The model under review builds one solid part; all positions refer to its coordinate system, in mm. A direction names the side the tool comes from. Round coordinates to 2 decimals unless told otherwise and drop trailing zeros. Loops run counter-clockwise (first coordinate to the right, second up) from the corner with the lowest first, then second, coordinate; pieces in that order, holes last. Notation, with made-up numbers: (59.25, -33) -> (112.25, -33) arc R24 cw to (112.25, -7) -> close; hole circle Ø7 at (13, -0.5). An arc over 180 degrees is marked (long way). Use a Markdown table: item, result. Add a question column.
1) Consider section A-A on x = 0. Give the boundary of the cut face in (y, z), plus the area to 3 significant figures.
2) Consider section C-C on z = -293.5. Give the boundary of the cut face in (x, y), plus the area to 3 significant figures.
3) For faces 1 (the cylindrical face through (23.517, -36.886, -300.533)), 2 (the flat face through (-4, -203.2, 100)), list the 3-axis set-ups (+Z, -Z, +X, -X, +Y, -Y) from which the entire face can be reached by the end or side of a thin tool; tool diameter is ignored.
4) Insertion check: pin 1 (12 mm diameter, centred on x = 137, y = 57, fed in from -Z). The pin has a flat end and moves straight along its axis. Give the tip position at first contact, or say it passes through.
5) Wall thickness on probe 1 along Z at (x, y) = (-12, 149); probe 2 along X at (y, z) = (-19.5, -450); probe 3 along Y at (x, z) = (-39.5, -228): over which ranges is each line inside the solid? List them lowest first.
6) Consider section D-D on y = 175. Give the boundary of the cut face in (x, z).
7) Consider section B-B on y = 0. Give the boundary of the cut face in (x, z).
from build123d import *

# Parameters (mm, degrees)
SKETCH_W     = 609.6
SKETCH_H     = 406.4
PAD_DEPTH    = 203.2
SKETCH001_R  = 43.745106
PAD001_DEPTH = 609.6


with BuildPart() as part:
    # Sketch → Pad (new body)
    with BuildSketch(Plane.XY):
        Rectangle(SKETCH_W, SKETCH_H)
    extrude(amount=PAD_DEPTH)

    # Sketch001 (on Face5 of Pad) → Pad001 (join)
    with BuildSketch(Plane(origin=(0, 0, 0), x_dir=(1, 0, 0), z_dir=(0, 0, -1))):
        Circle(SKETCH001_R)
    extrude(amount=PAD001_DEPTH)


solid = part.part
Result set:
| question | item | result |
|---|---|---|
| 1 | outline | (-203.2, 0) -> (-43.75, 0) -> (-43.75, -609.6) -> (43.75, -609.6) -> (43.75, 0) -> (203.2, 0) -> (203.2, 203.2) -> (-203.2, 203.2) -> close |
| 1 | area | 136,000 mm2 |
| 2 | outline | circle Ø87.49 at (0, 0) |
| 2 | area | 6,010 mm2 |
| 3 | face 1 | -Z |
| 3 | face 2 | +Z, -Z, +X, -X, -Y |
| 4 | pin 1 | z = 0 |
| 5 | probe 1 | 0 to 203.2 |
| 5 | probe 2 | -39.16 to 39.16 |
| 5 | probe 3 | -18.8 to 18.8 |
| 6 | outline | (-304.8, 0) -> (304.8, 0) -> (304.8, 203.2) -> (-304.8, 203.2) -> close |
| 7 | outline | (-304.8, 0) -> (-43.75, 0) -> (-43.75, -609.6) -> (43.75, -609.6) -> (43.75, 0) -> (304.8, 0) -> (304.8, 203.2) -> (-304.8, 203.2) -> close |
